Model file for the job. Use its own axes, mm. Face numbers are marked on the shaded views. Give positions to 0.01 mm unless a question says otherwise; leave off trailing zeros. Order: outer loops, then holes, each group sorted by start corner. A loop starts at its lowest first (then second) coordinate and runs counter-clockwise, first axis right, second up. Notation, with made-up numbers: (-39, 44) -> (12, 44) arc R29 ccw to (12, 65) -> close; hole circle Ø6 at (-4, -21). An arc over 180 degrees is marked (long way). Use CSV: the item, a comma, the result in double quotes. Start each with the question number.
1. Pull direction X, two halves, no side cores. Call the marked faces 1, 2, 3 and 4: released by +X, released by -X, zero draft, split by the parting line, or undercut.
2. Cut at B-B on y = -5.25. List the corners of the cut face in (x, z).
3. Wall check: line 1 (X direction, y = -10, z = 6); line 2 (Z direction, x = 7.5, y = -7); line 3 (Z direction, x = 5.75, y = -3.25). Give the ranges that are in metal, low to high. Write a range as from..to.
4. Cut at A-A on z = 6.25. List the corners of the cut face in (x, y) (3 decimals), then the cut area to 4 significant figures.
5. Cut at C-C on x = 11. List the corners of the cut face in (y, z), then the cut area to 3 significant figures.
6. Cut at D-D on x = 2.5. List the corners of the cut face in (y, z).
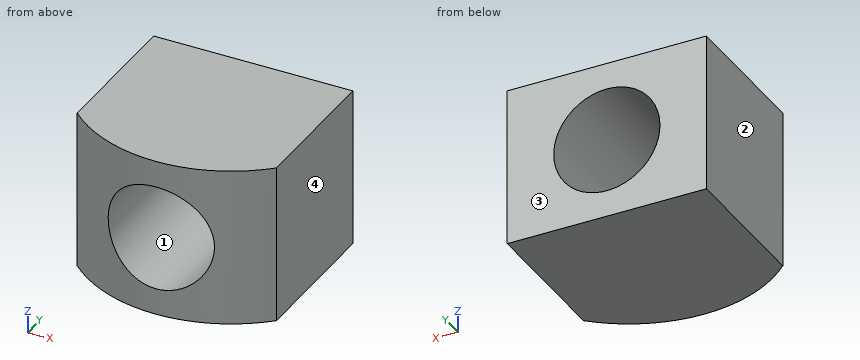
```python
from build123d import *

# Parameters (mm, degrees)
DODANIE_WYCI_GNI_CIE1_DEPTH = 12
SZKIC2_R                    = 4
WYTNIJ_WYCI_GNI_CIE1_DEPTH  = 21


with BuildPart() as part:
    # Szkic1 → Dodanie-wyciągnięcie1 (new body)
    with BuildSketch(Plane.XY):
        with BuildLine():
            Line((0, 0), (15, 0))
            Line((15, 0), (15, -11))
            ThreePointArc((15, -11), (7.5, -14), (0, -11))
            Line((0, -11), (0, 0))
        make_face()
    extrude(amount=DODANIE_WYCI_GNI_CIE1_DEPTH)

    # Szkic2 → Wytnij-wyciągnięcie1 (cut)
    with BuildSketch(Plane(origin=(0, 0, 0), x_dir=(1, 0, 0), z_dir=(0, 1, 0))):
        with Locations(Location((7.5, -6, 0), (0, 0, 270))):
            Circle(SZKIC2_R)
    extrude(amount=-WYTNIJ_WYCI_GNI_CIE1_DEPTH, mode=Mode.SUBTRACT)


solid = part.part
```
Verdict:
1,face 1,"undercut"
1,face 2,"released by -X"
1,face 3,"zero draft"
1,face 4,"released by +X"
2,outline,"(0, 0) -> (15, 0) -> (15, 12) -> (0, 12) -> close; hole circle Ø8 at (7.5, 6)"
3,line 1,"0..3.5, 11.5..15"
3,line 2,"0..2, 10..12"
3,line 3,"0..2.4, 9.6..12"
4,outline,"(0, -11) arc R10.875 ccw to (3.508, -13.241) -> (3.508, 0) -> (0, 0) -> close; (11.492, -13.241) arc R10.875 ccw to (15, -11) -> (15, 0) -> (11.492, 0) -> close"
4,area,"86.15 mm^2"
5,outline,"(-13.42, 0) -> (0, 0) -> (0, 4.06) -> (-13.42, 4.06) -> close; (-13.42, 7.94) -> (0, 7.94) -> (0, 12) -> (-13.42, 12) -> close"
5,area,"109 mm^2"
6,outline,"(-12.78, 0) -> (0, 0) -> (0, 12) -> (-12.78, 12) -> close"
